Check sheet for the drawn part. Datum: minimum x, y, z corner. Units: mm. A direction names the side the tool comes from. Give positions to 0.01 mm unless a question says otherwise; leave off trailing zeros. Loops run counter-clockwise (first coordinate to the right, second up) from the corner with the lowest first, then second, coordinate; pieces in that order, holes last. Notation, with made-up numbers: M 24,32.5 L 48,32.5 A29 cw 48,64.5 Z; hole C -7.5,-9.5 d6. An arc over 180 degrees is marked long. Write each question's results on one line, items separated by ' | '. Start each with the question number.
1. Draft check along X on the marked faces 3, 4, 5 and 6. Enter one of: pulls with the +X half, pulls with the -X half, needs draft (parallel to the pull), parting line crosses it, or undercut.
2. Sectioned sample at B-B on z = 46. Record the cut outline in (x, y), and give its area (3 significant figures).
3. Go/stop test with a flat-tipped pin: pin 1 (2 mm diameter, centred on x = 173, y = 53, fed in from -Z). Record where the tip stops, or that it passes through.
4. Sectioned sample at A-A on y = 14. Record the cut outline in (x, z).
5. Sectioned sample at C-C on x = 143.5. Record the cut outline in (y, z), and give its area (3 significant figures).
6. Material ranges on line 1 along X through (y, z) = (10.5, 64.5); line 2 along Z through (x, y) = (40, 101); line 3 along Y through (x, z) = (79, 94.5), recorded low to high.
7. Tool access check on the marked faces 1 and 2. Record the directions out of +Z, -Z, +X, -X, +Y, -Y that give a thin tool (end or side, any length) a straight path to the whole face; none if there is none.
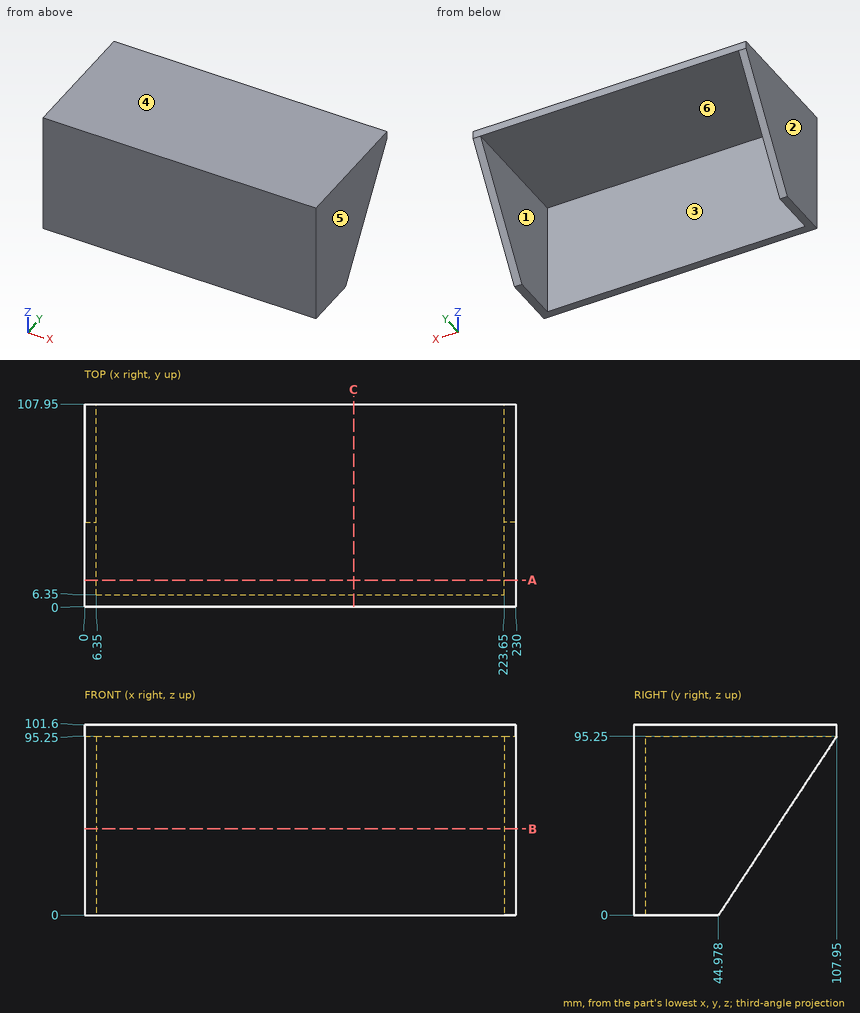
Output values:
1) face 3: undercut | face 4: needs draft | face 5: pulls with the +X half | face 6: undercut
2) outline: M 0,0 L 230,0 L 230,75.39 L 223.65,75.39 L 223.65,6.35 L 6.35,6.35 L 6.35,75.39 L 0,75.39 Z | area: 2,340 mm2
3) pin 1: z = 95.25
4) outline: M 0,0 L 6.35,0 L 6.35,95.25 L 223.65,95.25 L 223.65,0 L 230,0 L 230,101.6 L 0,101.6 Z
5) outline: M 0,0 L 6.35,0 L 6.35,95.25 L 107.95,95.25 L 107.95,101.6 L 0,101.6 Z | area: 1,290 mm2
6) line 1: 0 to 6.35, 223.65 to 230 | line 2: 95.25 to 101.6 | line 3: 0 to 6.35
7) face 1: -Z, +Y | face 2: +Z, -Z, -X, +Y, -Y
